Study the drawing (mm; zero at the part's minimum x, y, z) and answer. Coordinates: 2 decimals unless noted, no trailing zeros. Order: outer loops, then holes, each group sorted by start corner. A loop starts at its lowest first (then second) coordinate and runs counter-clockwise, first axis right, second up.
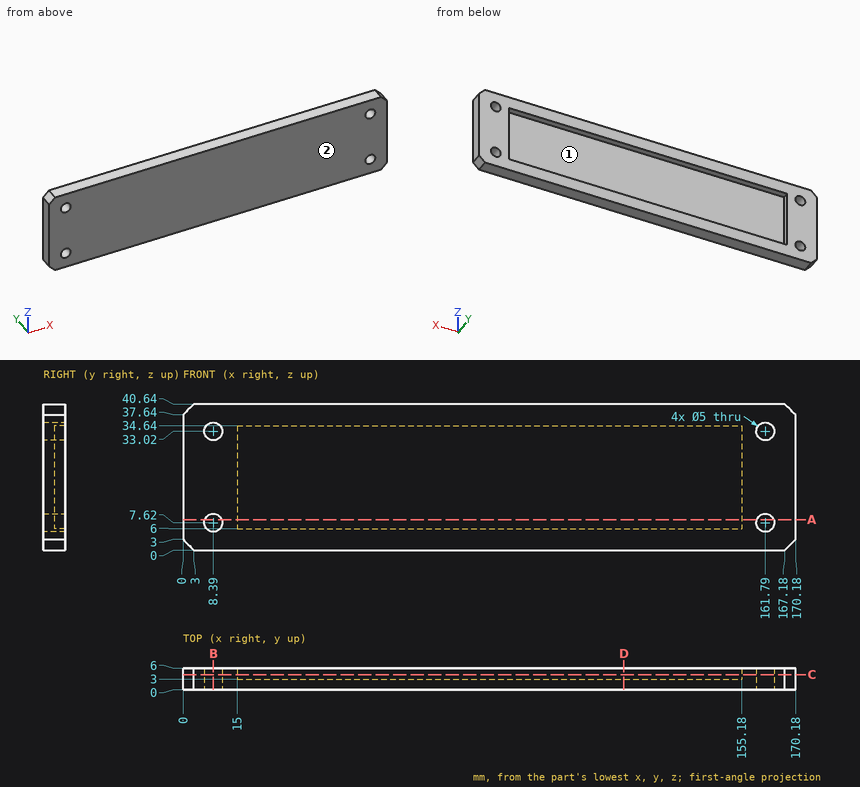
(1) The mould has two halves that part along X. Classify the marked faces 1 and 2: released by +X, released by -X, zero draft, split by the parting line, or undercut.
(2) Find section A-A (z = 8.5). Write down the section's boundary in (x, y).
(3) Find section C-C (y = 4.2). Write down the section's boundary in (x, z), and give its area (3 significant figures).
(4) Find section D-D (x = 122.5). Write down the section's boundary in (y, z).
(5) Consider line 1 (X direction, y = 3.65, z = 33.02); line 2 (X direction, y = 2.8, z = 7.5); line 3 (Z direction, x = 88.5, y = 3.25). Determine where each line is inside the solid, lowest interval first.
(6) Find section B-B (x = 8.39). Write down the section's boundary in (y, z).
Findings below:
1. face 1: undercut
1. face 2: zero draft
2. outline: (0, 0) - (6.05, 0) - (6.05, 6) - (0, 6) - close; (10.73, 0) - (159.45, 0) - (159.45, 6) - (155.18, 6) - (155.18, 3) - (15, 3) - (15, 6) - (10.73, 6) - close; (164.13, 0) - (170.18, 0) - (170.18, 6) - (164.13, 6) - close
3. outline: (0, 3) - (3, 0) - (167.18, 0) - (170.18, 3) - (170.18, 37.64) - (167.18, 40.64) - (3, 40.64) - (0, 37.64) - close; hole circle Ø5 at (8.39, 7.62); hole circle Ø5 at (8.39, 33.02); hole (15, 6) - (155.18, 6) - (155.18, 34.64) - (15, 34.64) - close; hole circle Ø5 at (161.79, 7.62); hole circle Ø5 at (161.79, 33.02)
3. area: 2,800 mm2
4. outline: (0, 0) - (6, 0) - (6, 6) - (3, 6) - (3, 34.64) - (6, 34.64) - (6, 40.64) - (0, 40.64) - close
5. line 1: x = 0 to 5.89, 10.89 to 15, 155.18 to 159.29, 164.29 to 170.18
5. line 2: x = 0 to 5.89, 10.89 to 159.29, 164.29 to 170.18
5. line 3: z = 0 to 6, 34.64 to 40.64
6. outline: (0, 0) - (6, 0) - (6, 5.12) - (0, 5.12) - close; (0, 10.12) - (6, 10.12) - (6, 30.52) - (0, 30.52) - close; (0, 35.52) - (6, 35.52) - (6, 40.64) - (0, 40.64) - close
